from build123d import *

# Parameters (mm, degrees)
ESQUISSE1_W        = 840
ESQUISSE1_H        = 1100
BOSS_EXTRU_1_DEPTH = 30
ESQUISSE2_W        = 840
ESQUISSE2_H        = 1100
ESQUISSE2_W_2      = 786
ESQUISSE2_H_2      = 1046
BOSS_EXTRU_2_DEPTH = 1900
ESQUISSE4_W        = 786
ESQUISSE4_H        = 27
BOSS_EXTRU_3_DEPTH = 540


with BuildPart() as part:
    # Esquisse1 → Boss.-Extru.1 (new body)
    with BuildSketch(Plane.XY):
        with Locations((420, 550)):
            Rectangle(ESQUISSE1_W, ESQUISSE1_H)
    extrude(amount=BOSS_EXTRU_1_DEPTH)

    # Esquisse2 → Boss.-Extru.2 (add)
    with BuildSketch(Plane.XY.offset(30)):
        with Locations((420, 550)):
            Rectangle(ESQUISSE2_W, ESQUISSE2_H)
        with Locations((420, 550)):
            Rectangle(ESQUISSE2_W_2, ESQUISSE2_H_2, mode=Mode.SUBTRACT)
    extrude(amount=BOSS_EXTRU_2_DEPTH)

    # Esquisse4 → Boss.-Extru.3 (add)
    with BuildSketch(Plane(origin=(0, 1100, 0), x_dir=(1, 0, 0), z_dir=(0, 1, 0))):
        with Locations((420, -443.5)):
            Rectangle(ESQUISSE4_W, ESQUISSE4_H)
    extrude(amount=-BOSS_EXTRU_3_DEPTH)


solid = part.part
Here's how the part is built. I have some questions about the finished solid (model axes, mm). A direction names the side the tool comes from. Give positions to 0.01 mm unless a question says otherwise; leave off trailing zeros. Order: outer loops, then holes, each group sorted by start corner. A loop starts at its lowest first (then second) coordinate and runs counter-clockwise, first axis right, second up. Notation, with made-up numbers: (75, -17.5) -> (119, -17.5) arc R6 cw to (119, -9.5) -> close; hole circle Ø4 at (4, 67). An arc over 180 degrees is marked (long way). Use a Markdown table: item, result. Add a question column.
Item 1: Imagine slicing it at C-C on x = 703. Please give me the cut outline in (y, z), plus the area to 3 significant figures.
Item 2: Imagine slicing it at B-B on z = 392.5. Please give me the cut outline in (x, y).
Item 3: I need wall thicknesses on line 1 (X direction, y = 349, z = 1113.5); line 2 (Y direction, x = 444.5, z = 1457); line 3 (Z direction, x = 598.5, y = 667.5). Which ranges of each line are inside material? Lowest first, please.
Item 4: Imagine slicing it at D-D on y = 168. Please give me the cut outline in (x, z).
Item 5: Imagine slicing it at A-A on y = 896. Please give me the cut outline in (x, z), plus the area to 3 significant figures.
Item 6: If we mould it in two halves opening along Z, with no side actions, what happens to faces 4 (the face through (414, 1073, 1183)), 5 (the face through (414, 820, 430)), 6 (the face through (414, 558, 0))? For each: pulls with the +Z half, pulls with the -Z half, needs draft (parallel to the pull), parting line crosses it, or undercut.
Item 7: Will this pin go through, and if not, where does the flat tip stop? pin 1 (12 mm diameter, centred on x = 630, y = 151, fed in from +Z).
Item 8: For faces 1 (the face through (414, 0, 951)), 2 (the face through (414, 1073, 227)), 3 (the face through (414, 27, 967)), which set-ups out of +Z, -Z, +X, -X, +Y, -Y let a thin tool reach every point of the face, with its end or its side?
Data:
| question | item | result |
|---|---|---|
| 1 | outline | (0, 0) -> (1100, 0) -> (1100, 1930) -> (1073, 1930) -> (1073, 457) -> (560, 457) -> (560, 430) -> (1073, 430) -> (1073, 30) -> (27, 30) -> (27, 1930) -> (0, 1930) -> close |
| 1 | area | 149,000 mm² |
| 2 | outline | (0, 0) -> (840, 0) -> (840, 1100) -> (0, 1100) -> close; hole (27, 27) -> (813, 27) -> (813, 1073) -> (27, 1073) -> close |
| 3 | line 1 | x = 0 to 27, 813 to 840 |
| 3 | line 2 | y = 0 to 27, 1073 to 1100 |
| 3 | line 3 | z = 0 to 30, 430 to 457 |
| 4 | outline | (0, 0) -> (840, 0) -> (840, 1930) -> (813, 1930) -> (813, 30) -> (27, 30) -> (27, 1930) -> (0, 1930) -> close |
| 5 | outline | (0, 0) -> (840, 0) -> (840, 1930) -> (813, 1930) -> (813, 457) -> (27, 457) -> (27, 1930) -> (0, 1930) -> close; hole (27, 30) -> (813, 30) -> (813, 430) -> (27, 430) -> close |
| 5 | area | 149,000 mm² |
| 6 | face 4 | needs draft |
| 6 | face 5 | undercut |
| 6 | face 6 | pulls with the -Z half |
| 7 | pin 1 | stops at z = 30 |
| 8 | face 1 | +Z, -Z, +X, -X, -Y |
| 8 | face 2 | none |
| 8 | face 3 | +Z |
